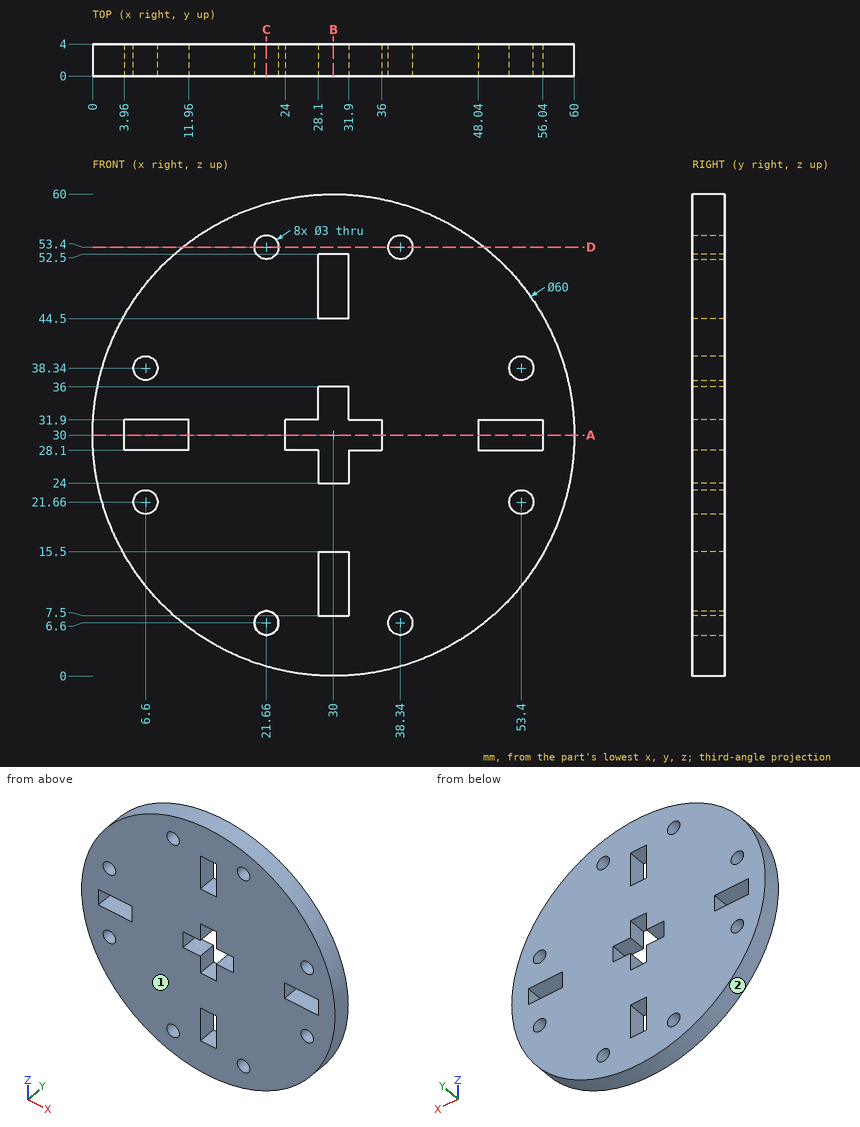
Verification items for this drawing (mm, ordinates from the low corner). Coordinates: 2 decimals unless noted, no trailing zeros. Loops run counter-clockwise (first coordinate to the right, second up) from the corner with the lowest first, then second, coordinate; pieces in that order, holes last.
Item 1: Thickness scan on line 1 (Z direction, x = 38.34, y = 2.6); line 2 (Z direction, x = 38, y = 2.2). Record the ranges inside material, lowest first.
Item 2: Release check for a two-part mould opening along Z. For the marked faces 1 and 2 record: released by +Z, released by -Z, zero draft, split by the parting line, or undercut.
Item 3: Sectioned sample at A-A, the plane z = 30. Record the boundary of the cut face in (x, y), then the cut area to 3 significant figures.
Item 4: Go/stop test with flat-tipped pins: pin 1 Ø1.2 at (y, z) = (1.5, 49.5) entering from -X; pin 2 Ø1.5 at (x, y) = (29, 3) entering from +Z; pin 3 Ø1.8 at (x, z) = (38.34, 53.4) entering from +Y; pin 4 Ø1.1 at (x, y) = (30, 2.5) entering from -Z. Record where each tip stops, or that it passes through.
Item 5: Sectioned sample at C-C, the plane x = 21.66. Record the boundary of the cut face in (y, z), then the cut area to 3 significant figures.
Item 6: Sectioned sample at B-B, the plane x = 30. Record the boundary of the cut face in (y, z).
Item 7: Sectioned sample at D-D, the plane z = 53.4. Record the boundary of the cut face in (x, y), then the cut area to 3 significant figures.
Check result:
1. line 1: z = 1.18 to 5.1, 8.1 to 51.9, 54.9 to 58.82
1. line 2: z = 1.09 to 5.14, 8.06 to 51.94, 54.86 to 58.91
2. face 1: zero draft
2. face 2: split by the parting line
3. outline: (0, 0) - (3.96, 0) - (3.96, 4) - (0, 4) - close; (11.96, 0) - (24, 0) - (24, 4) - (11.96, 4) - close; (36, 0) - (48.04, 0) - (48.04, 4) - (36, 4) - close; (56.04, 0) - (60, 0) - (60, 4) - (56.04, 4) - close
3. area: 128 mm2
4. pin 1: stops at x = 6.7
4. pin 2: stops at z = 60
4. pin 3: passes through
4. pin 4: stops at z = 0
5. outline: (0, 1.18) - (4, 1.18) - (4, 5.1) - (0, 5.1) - close; (0, 8.1) - (4, 8.1) - (4, 51.9) - (0, 51.9) - close; (0, 54.9) - (4, 54.9) - (4, 58.82) - (0, 58.82) - close
5. area: 207 mm2
6. outline: (0, 0) - (4, 0) - (4, 7.5) - (0, 7.5) - close; (0, 15.5) - (4, 15.5) - (4, 24) - (0, 24) - close; (0, 36) - (4, 36) - (4, 44.5) - (0, 44.5) - close; (0, 52.5) - (4, 52.5) - (4, 60) - (0, 60) - close
7. outline: (11.23, 0) - (20.16, 0) - (20.16, 4) - (11.23, 4) - close; (23.16, 0) - (36.84, 0) - (36.84, 4) - (23.16, 4) - close; (39.84, 0) - (48.77, 0) - (48.77, 4) - (39.84, 4) - close
7. area: 126 mm2
